from build123d import *

# Parameters (mm, degrees)
BOSS_EXTRUDE1_DEPTH = 8
SKETCH2_R           = 2.2500000000000058
BOSS_EXTRUDE2_DEPTH = 5.125
FILLET1_R           = 10
FILLET5_R           = 5
FILLET6_R           = 2
SKETCH5_R           = 2.749999999999998
CUT_EXTRUDE1_DEPTH  = 29.057975693196408
SKETCH5_3_R         = 5.000000000000001
SKETCH5_3_R_2       = 2.749999999999998
CUT_EXTRUDE2_DEPTH  = 3
CUT_EXTRUDE3_DEPTH  = 31.095940340849967
FILLET8_R           = 8
FILLET11_R          = 0.75


# Some blends are built 0.0001 mm under size
with BuildPart() as part:
    # Sketch1 → Boss-Extrude1 (new body)
    with BuildSketch(Plane.XY):
        Polygon((-9, 17.500000000000004), (9, 17.500000000000004), (9.000000000000004, -17.499999999999996), (-8.999999999999996, -17.499999999999996), align=None)
    extrude(amount=BOSS_EXTRUDE1_DEPTH)

    # Sketch2 → Boss-Extrude2 (add, symmetric)
    with BuildSketch(Plane(origin=(0, 0, 0), x_dir=(0, 0, -1), z_dir=(1, 0, 0))):
        Polygon((0, 17.500000000000004), (20, 17.500000000000007), (20.000000000000007, -2.499999999999992), (2.14e-15, -2.499999999999992), align=None)
        with Locations((13.000000000000002, 7.500000000000007)):
            Circle(SKETCH2_R, mode=Mode.SUBTRACT)
    extrude(amount=BOSS_EXTRUDE2_DEPTH, both=True)

    # Fillet1
    fillet1_edges = [part.edges().sort_by_distance(p)[0] for p in [
        (0, 17.500000000000007, -20),
        (0, -2.499999999999992, -20.000000000000007),
    ]]
    fillet(fillet1_edges, radius=FILLET1_R - 0.0001)  # a hair under: the kernel refuses the full size

    # Fillet5
    fillet5_edges = [part.edges().sort_by_distance(p)[0] for p in [
        (9.000000000000004, -17.499999999999996, 4),
        (-8.999999999999996, -17.499999999999996, 4),
    ]]
    fillet(fillet5_edges, radius=FILLET5_R)

    # Fillet6
    fillet6_edges = [part.edges().sort_by_distance(p)[0] for p in [
        (-9, 17.500000000000004, 4),
        (9, 17.500000000000004, 4),
    ]]
    fillet(fillet6_edges, radius=FILLET6_R)

    # Sketch5 → Cut-Extrude1 (cut, through all)
    with BuildSketch(Plane(origin=(0, 0, 0), x_dir=(-1, 0, 0), z_dir=(0, 0, -1))):
        with Locations((0, -8.75)):
            Circle(SKETCH5_R)
    extrude(amount=-CUT_EXTRUDE1_DEPTH, mode=Mode.SUBTRACT)

    # Sketch5<3> → Cut-Extrude2 (cut)
    with BuildSketch(Plane(origin=(0, 0, 0), x_dir=(-1, 0, 0), z_dir=(0, 0, -1))):
        with Locations((0, -8.75)):
            Circle(SKETCH5_3_R)
        with Locations((0, -8.75)):
            Circle(SKETCH5_3_R_2, mode=Mode.SUBTRACT)
    extrude(amount=-CUT_EXTRUDE2_DEPTH, mode=Mode.SUBTRACT)

    # Sketch6 → Cut-Extrude3 (cut, through all)
    with BuildSketch(Plane(origin=(5.125, 0, 0), x_dir=(0, 0, -1), z_dir=(1, 0, 0))):
        Polygon((0, 17.500000000000004), (20, 17.500000000000004), (20.000000000000004, 15.250000000000005), (2.8e-16, 15.250000000000005), align=None)
        Polygon((19.999999999999996, -2.499999999999992), (20.000000000000004, -0.24999999999998807), (7.21e-15, -0.24999999999999156), (6.94e-15, -2.499999999999992), align=None)
    extrude(amount=-CUT_EXTRUDE3_DEPTH, mode=Mode.SUBTRACT)

    # Fillet8
    # the kernel refuses this fillet: 8 mm, written as the material it takes off along each edge
    with BuildSketch(Plane(origin=(29.35923701875709, -0.2499999999999887, -16.31967672633224), x_dir=(0, -1.5e-16, 1), z_dir=(-1, 0, 0))) as fillet8_piece_1:
        with BuildLine():
            CenterArc((4.335351436704053, 8), FILLET8_R, 172.8217708442513, 97.17822915574868)
            Line((-3.6019465867097984, 8.99964998249916), (-4.395676389051184, 9.099614980749076))
            ThreePointArc((-4.395676389051184, 9.099614980749076), (-4.480323273667765, 7.750099999999992), (-0.5055711938185182, -0.6199981999819997))
            Line((-0.5055711938185182, -0.6199981999819997), (1.2e-16, -0.8))
            Line((1.2e-16, -0.8), (4.335351436704052, -0.8))
            Line((4.335351436704052, -0.8), (4.335351436704052, 0))
        make_face()
    extrude(amount=58.718474037514184, mode=Mode.SUBTRACT)
    with BuildSketch(Plane(origin=(29.35923701875702, 15.250000000000005, -16.31967672633223), x_dir=(0, -0.9284024472828977, -0.37157623158529146), z_dir=(-1, 0, 0))) as fillet8_piece_2:
        with BuildLine():
            CenterArc((5.816306028814807, 6.9975607363498025), FILLET8_R, 201.81286045411787, 97.17822915574845)
            Line((-1.610913549448369, 4.024950883667459), (-2.3536355072746873, 3.727689898399224))
            Line((-2.3536355072746873, 3.727689898399224), (-0.7427219578263171, -0.29726098526823275))
            Line((-0.7427219578263171, -0.29726098526823275), (-0.38774960717711915, -0.6997501283558207))
            ThreePointArc((-0.38774960717711915, -0.6997501283558207), (8.859993445000528, -1.2797901394825208), (10.081433685371605, -0.6997560736349794))
            Line((10.081433685371605, -0.6997560736349794), (9.693694807502807, 5.1e-16))
        make_face()
    extrude(amount=58.71847403751404, mode=Mode.SUBTRACT)

    # Fillet11
    fillet11_edges = [part.edges().sort_by_distance(p)[0] for p in [
        (5.125, -0.2499999999999905, -5.9921626448140035),
        (-5.125, -0.24999999999999029, -5.9921626448140035),
        (5.125, 12.994562646523407, -17.552089652471594),
        (5.125, 2.00543735344751, -17.5520896524431),
        (-5.125, 12.994562646523407, -17.552089652471594),
        (-5.125, 2.00543735344751, -17.5520896524431),
        (0, 17.500000000000004, 0),
        (9.000000000000002, 1.5000000000000036, 0),
        (9.000000000000002, 1.5000000000000036, 8),
        (3.55e-15, -17.499999999999996, 0),
        (-7.535533905932736, -16.035533905932734, 0),
        (7.535533905932741, -16.035533905932734, 0),
        (3.55e-15, -17.499999999999996, 8),
        (-7.535533905932736, -16.035533905932734, 8),
        (7.535533905932741, -16.035533905932734, 8),
        (-8.999999999999998, 1.5000000000000036, 0),
        (-8.999999999999998, 1.5000000000000036, 8),
        (8.414213562373096, 16.9142135623731, 0),
        (-8.414213562373096, 16.9142135623731, 0),
        (0, 17.500000000000004, 8),
        (8.414213562373096, 16.9142135623731, 8),
        (-8.414213562373096, 16.9142135623731, 8),
        (-5.125, 7.500000000000006, -1.07e-15),
        (5.125, 7.500000000000006, -1.07e-15),
        (-5.125, 15.250000000000005, -5.992162644814096),
        (0, 15.250000000000005, -2.8e-16),
        (5.125, 15.250000000000005, -5.992162644814096),
        (0, -0.24999999999999156, -7.21e-15),
    ]]
    fillet(fillet11_edges, radius=FILLET11_R)


solid = part.part
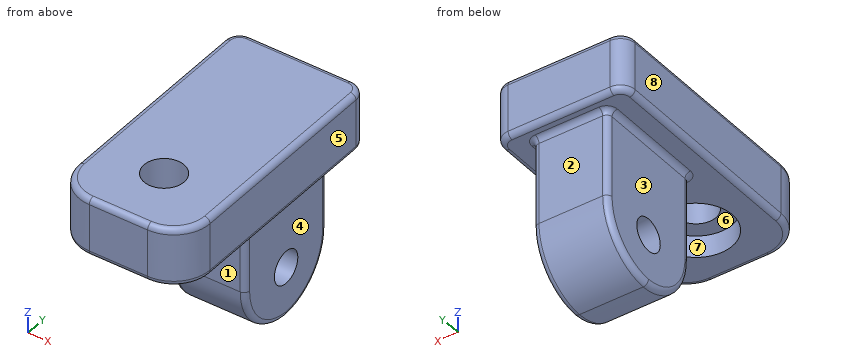
Input: part model. Units: mm. Frame: model coordinates. Face numbers are marked on the shaded views. A direction names the side the tool comes from. Give positions to 0.01 mm unless a question says otherwise; leave off trailing zeros. Write each loop counter-clockwise with the first axis right and the second up, starting at its lowest first coordinate (ties: lowest second). Pieces come first, ordered by that corner, then holes. Notation, with made-up numbers: (57.5, 60) -> (106.5, 60) arc R13 ccw to (106.5, 74) -> close; hole circle Ø4 at (34.5, 11). An arc over 180 degrees is marked (long way). Use one line per item in the form item = value. Start each with the question number.
1) Ray query, probe 1 along Y at (x, z) = (0, 5.65); probe 2 along Z at (x, y) = (2.75, -12.5); probe 3 along X at (y, z) = (1, -2.25) (3 decimals). Return the intervals inside material, ascending. Write a range as from..to.
2) Section query B-B on x = 0. Return the cut outline in (y, z).
3) Pin query (flat end, axial travel): pin 1 (2.5 mm diameter, centred on x = -1, z = -5, fed in from +Y); pin 2 (8 mm diameter, centred on x = 0, y = -8.75, fed in from +Z); pin 3 (4.5 mm diameter, centred on x = -0.5, z = -6.5, fed in from -Y); pin 4 (4.5 mm diameter, centred on x = 0, y = -8.75, fed in from +Z). Return the tip coordinate at first contact, or that it passes through.
4) Section query A-A on y = -8.75. Return the cut outline in (x, z).
5) Set-up query: the marked faces 1, 2, 3 and 4. Return all of +Z, -Z, +X, -X, +Y, -Y with unobstructed straight access to the full face (end or side cutting, diameter ignored); none if empty.
6) Draft query along X for the marked faces 5, 6, 7 and 8. Return one class per face: pulls with the +X half, pulls with the -X half, needs draft (parallel to the pull), parting line crosses it, or undercut.
Outcome:
q1.probe_1 = -17.5..-11.5, -6..17.5
q1.probe_2 = 3..8
q1.probe_3 = -5.125..5.125
q2.outline = (-17.5, 0.75) arc R0.75 ccw to (-16.75, 0) -> (-13.75, 0) -> (-13.75, 3) -> (-11.5, 3) -> (-11.5, 8) -> (-16.75, 8) arc R0.75 ccw to (-17.5, 7.25) -> close; (-6, 3) -> (-3.75, 3) -> (-3.75, 0) -> (-1, 0) arc R0.75 cw to (-0.25, -0.75) -> (-0.25, -11.98) arc R8 ccw to (7.5, -19.98) arc R8 ccw to (15.25, -11.98) -> (15.25, -0.75) arc R0.75 cw to (16, 0) -> (16.75, 0) arc R0.75 ccw to (17.5, 0.75) -> (17.5, 7.25) arc R0.75 ccw to (16.75, 8) -> (-6, 8) -> close; hole circle Ø4.5 at (7.5, -13)
q3.pin_1 = 15.25
q3.pin_2 = 8
q3.pin_3 = -0.25
q3.pin_4 = through
q4.outline = (-9, 0.75) arc R0.75 ccw to (-8.25, 0) -> (-5, 0) -> (-5, 3) -> (-2.75, 3) -> (-2.75, 8) -> (-8.25, 8) arc R0.75 ccw to (-9, 7.25) -> close; (2.75, 3) -> (5, 3) -> (5, 0) -> (8.25, 0) arc R0.75 ccw to (9, 0.75) -> (9, 7.25) arc R0.75 ccw to (8.25, 8) -> (2.75, 8) -> close
q5.face_1 = -Z, +X, -X, -Y
q5.face_2 = -Z, +X, -X, +Y
q5.face_3 = -Z, -X, +Y, -Y
q5.face_4 = -Z, +X, +Y, -Y
q6.face_5 = pulls with the +X half
q6.face_6 = undercut
q6.face_7 = undercut
q6.face_8 = pulls with the -X half
